from build123d import *

# Parameters (mm, degrees)
SKICA1_W                  = 191
SKICA1_H                  = 175
P_IDAT_VYSUNUT_M1_DEPTH   = 3
SKICA13_W                 = 25
SKICA13_H                 = 3
SKICA13_W_2               = 8
P_IDAT_VYSUNUT_M5_DEPTH   = 3
SKICA14_W                 = 3
SKICA14_H                 = 5
ODEBRAT_VYSUNUT_M7_DEPTH  = 132.60357138
SKICA15_W                 = 3
SKICA15_H                 = 25
ODEBRAT_VYSUNUT_M8_DEPTH  = 132.60357138
SKICA16_W                 = 3
SKICA16_H                 = 5
ODEBRAT_VYSUNUT_M9_DEPTH  = 132.60357138
SKICA4_R                  = 2.15
SKICA4_R_2                = 60
ODEBRAT_VYSUNUT_M5_DEPTH  = 132.60357138
SKICA5_R                  = 9.5
ODEBRAT_VYSUNUT_M6_DEPTH  = 132.60357138
SKICA17_R                 = 1.5
SKICA17_W                 = 13.5
SKICA17_H                 = 6.5
ODEBRAT_VYSUNUT_M10_DEPTH = 132.60357138


with BuildPart() as part:
    # Skica1 → Přidat vysunutím1 (new body)
    with BuildSketch(Plane(origin=(0, 0, 0), x_dir=(1, 0, 0), z_dir=(0, 1, 0))):
        Rectangle(SKICA1_W, SKICA1_H)
    extrude(amount=P_IDAT_VYSUNUT_M1_DEPTH)

    # Skica13 → Přidat vysunutím5 (add)
    with BuildSketch(Plane(origin=(0, 0, 0), x_dir=(1, 0, 0), z_dir=(0, 1, 0))):
        with Locations((-50, 89)):
            Rectangle(SKICA13_W, SKICA13_H)
        with Locations((0, 89)):
            Rectangle(SKICA13_W, SKICA13_H)
        with Locations((50, 89)):
            Rectangle(SKICA13_W, SKICA13_H)
        with Locations((50, -89)):
            Rectangle(SKICA13_W, SKICA13_H)
        with Locations((0, -89)):
            Rectangle(SKICA13_W, SKICA13_H)
        with Locations((-50, -89)):
            Rectangle(SKICA13_W, SKICA13_H)
        with Locations((-91.5, 89)):
            Rectangle(SKICA13_W_2, SKICA13_H)
        with Locations((91.5, -89)):
            Rectangle(SKICA13_W_2, SKICA13_H)
        with Locations((91.5, 89)):
            Rectangle(SKICA13_W_2, SKICA13_H)
        with Locations((-91.5, -89)):
            Rectangle(SKICA13_W_2, SKICA13_H)
    extrude(amount=P_IDAT_VYSUNUT_M5_DEPTH)

    # Skica14 → Odebrat vysunutím7 (cut, through all)
    with BuildSketch(Plane(origin=(0, 0, 0), x_dir=(1, 0, 0), z_dir=(0, 1, 0))):
        with Locations((87, 80)):
            Rectangle(SKICA14_W, SKICA14_H)
        with Locations((0, 80)):
            Rectangle(SKICA14_W, SKICA14_H)
        with Locations((-87, 80)):
            Rectangle(SKICA14_W, SKICA14_H)
    extrude(amount=ODEBRAT_VYSUNUT_M7_DEPTH, mode=Mode.SUBTRACT)

    # Skica15 → Odebrat vysunutím8 (cut, through all)
    with BuildSketch(Plane(origin=(0, 0, 0), x_dir=(1, 0, 0), z_dir=(0, 1, 0))):
        with Locations((-90, 50)):
            Rectangle(SKICA15_W, SKICA15_H)
        with Locations((-90, 0)):
            Rectangle(SKICA15_W, SKICA15_H)
        with Locations((-90, -50)):
            Rectangle(SKICA15_W, SKICA15_H)
        with Locations((90, -50)):
            Rectangle(SKICA15_W, SKICA15_H)
        with Locations((90, 0)):
            Rectangle(SKICA15_W, SKICA15_H)
        with Locations((90, 50)):
            Rectangle(SKICA15_W, SKICA15_H)
    extrude(amount=ODEBRAT_VYSUNUT_M8_DEPTH, mode=Mode.SUBTRACT)

    # Skica16 → Odebrat vysunutím9 (cut, through all)
    with BuildSketch(Plane(origin=(0, 0, 0), x_dir=(1, 0, 0), z_dir=(0, 1, 0))):
        with Locations((-66.5, -5)):
            Rectangle(SKICA16_W, SKICA16_H)
        with Locations((-66.5, -15)):
            Rectangle(SKICA16_W, SKICA16_H)
        with Locations((66.5, -15)):
            Rectangle(SKICA16_W, SKICA16_H)
        with Locations((66.5, -5)):
            Rectangle(SKICA16_W, SKICA16_H)
    extrude(amount=ODEBRAT_VYSUNUT_M9_DEPTH, mode=Mode.SUBTRACT)

    # Skica4 → Odebrat vysunutím5 (cut, through all)
    with BuildSketch(Plane(origin=(0, 0, 0), x_dir=(1, 0, 0), z_dir=(0, 1, 0))):
        with Locations(Location((-52.5, -62.5, 0), (0, 0, 90))):
            Circle(SKICA4_R)
        with Locations(Location((52.5, 42.5, 0), (0, 0, 90))):
            Circle(SKICA4_R)
        with Locations(Location((0, -10, 0), (0, 0, 90))):
            Circle(SKICA4_R_2)
        with Locations(Location((-52.5, 42.5, 0), (0, 0, 90))):
            Circle(SKICA4_R)
        with Locations(Location((52.5, -62.5, 0), (0, 0, 90))):
            Circle(SKICA4_R)
    extrude(amount=ODEBRAT_VYSUNUT_M5_DEPTH, mode=Mode.SUBTRACT)

    # Skica5 → Odebrat vysunutím6 (cut, through all)
    with BuildSketch(Plane(origin=(0, 0, 0), x_dir=(1, 0, 0), z_dir=(0, 1, 0))):
        with Locations(Location((55.5, 67.5, 0), (0, 0, 90))):
            Circle(SKICA5_R)
    extrude(amount=ODEBRAT_VYSUNUT_M6_DEPTH, mode=Mode.SUBTRACT)

    # Skica17 → Odebrat vysunutím10 (cut, through all)
    with BuildSketch(Plane(origin=(0, 0, 0), x_dir=(1, 0, 0), z_dir=(0, 1, 0))):
        with Locations(Location((-78, 67.5, 0), (0, 0, 90))):
            Circle(SKICA17_R)
        with Locations(Location((-49, 67.5, 0), (0, 0, 90))):
            Circle(SKICA17_R)
        with Locations(Location((-38, 67.5, 0), (0, 0, 90))):
            Circle(SKICA17_R)
        with Locations(Location((-9, 67.5, 0), (0, 0, 90))):
            Circle(SKICA17_R)
        with Locations((-63.5, 67.5)):
            Rectangle(SKICA17_W, SKICA17_H)
        with Locations((-23.5, 67.5)):
            Rectangle(SKICA17_W, SKICA17_H)
    extrude(amount=ODEBRAT_VYSUNUT_M10_DEPTH, mode=Mode.SUBTRACT)


solid = part.part
The model under review builds one solid part; all positions refer to its coordinate system, in mm. Coordinates: 2 decimals unless noted, no trailing zeros. Loops run counter-clockwise (first coordinate to the right, second up) from the corner with the lowest first, then second, coordinate; pieces in that order, holes last. Notation, with made-up numbers: M 46,-35 L 78,-35 A14 cw 78,-22 Z; hole C 74,5.5 d10. An arc over 180 degrees is marked long. Put each result on its own line as item: value. Start each with the question number.
Q1. The part is to be moulded in two halves that separate along Z. For faces 1 (the flat face through (41, 3, -41)), 2 (the cylindrical face through (50.69, 1.48, -43.66)), say which applies: +Z half, -Z half, draft (parallel to the pull), parting line (faces both ways), or undercut.
Q2. Add section C-C (z = 45). Write out the cut boundary in (x, y).
Q3. Add section A-A (z = -54.5). Write out the cut boundary in (x, y), and give its area (3 significant figures).
Q4. Clearance check with flat-ended pins moving along their axes: pin 1 (0.9 mm diameter, centred on x = 86.5, y = 1.5, fed in from +Z); pin 2 (1 mm diameter, centred on x = -62, z = 21.5, fed in from -Y); pin 3 (1.5 mm diameter, centred on x = 69.5, y = 2, fed in from -Z); pin 4 (2 mm diameter, centred on x = -59.5, z = -68.5, fed in from +Y). State where each tip first meets the part, or that it passes through.
Q5. Add section B-B (x = 52.5). Write out the cut boundary in (y, z).
Q6. Add section D-D (y = 2.35). Count the separate pieces of the cut face and the enclosed holes in it, and give its area (3 significant figures).
Q7. Wall thickness on line 1 (X direction, y = 2, z = 10); line 2 (Z direction, x = 54, y = 0.7); line 3 (Z direction, x = -24, y = 2.45): over which ranges is each line inside the solid? List them lowest first.
Answers:
1. face 1: draft
1. face 2: undercut
2. outline: M -95.5,0 L -91.5,0 L -91.5,3 L -95.5,3 Z; M -88.5,0 L -48.73,0 L -48.73,3 L -88.5,3 Z; M 48.73,0 L 88.5,0 L 88.5,3 L 48.73,3 Z; M 91.5,0 L 95.5,0 L 95.5,3 L 91.5,3 Z
3. outline: M -95.5,0 L -91.5,0 L -91.5,3 L -95.5,3 Z; M -88.5,0 L 88.5,0 L 88.5,3 L -88.5,3 Z; M 91.5,0 L 95.5,0 L 95.5,3 L 91.5,3 Z
3. area: 555 mm^2
4. pin 1: stops at z = 87.5
4. pin 2: stops at y = 0
4. pin 3: stops at z = -87.5
4. pin 4: passes through
5. outline: M 0,-90.5 L 3,-90.5 L 3,-76.51 L 0,-76.51 Z; M 0,-58.49 L 3,-58.49 L 3,-44.65 L 0,-44.65 Z; M 0,-40.35 L 3,-40.35 L 3,-19.05 L 0,-19.05 Z; M 0,39.05 L 3,39.05 L 3,60.35 L 0,60.35 Z; M 0,64.65 L 3,64.65 L 3,90.5 L 0,90.5 Z
6. separate pieces: 1
6. enclosed holes: 25
6. area: 21,600 mm^2
7. line 1: x = -95.5 to -91.5, -88.5 to -60, 60 to 88.5, 91.5 to 95.5
7. line 2: z = -90.5 to -76.88, -58.12 to -44.04, -40.96 to -16.15, 36.15 to 60.96, 64.04 to 90.5
7. line 3: z = -87.5 to -70.75, -64.25 to -44.99, 64.99 to 87.5
